Could you check a few things on this drawing? It's one solid part, dimensions in mm from its lowest x, y, z. Give positions to 0.01 mm unless a question says otherwise; leave off trailing zeros. Order: outer loops, then holes, each group sorted by start corner. A loop starts at its lowest first (then second) coordinate and runs counter-clockwise, first axis right, second up. Notation, with made-up numbers: M 16,36 L 43,36 A10 ccw 43,45 Z; hole C 26.5,20 d10. An arc over 180 degrees is marked long. Use one line per item in the form item = value.
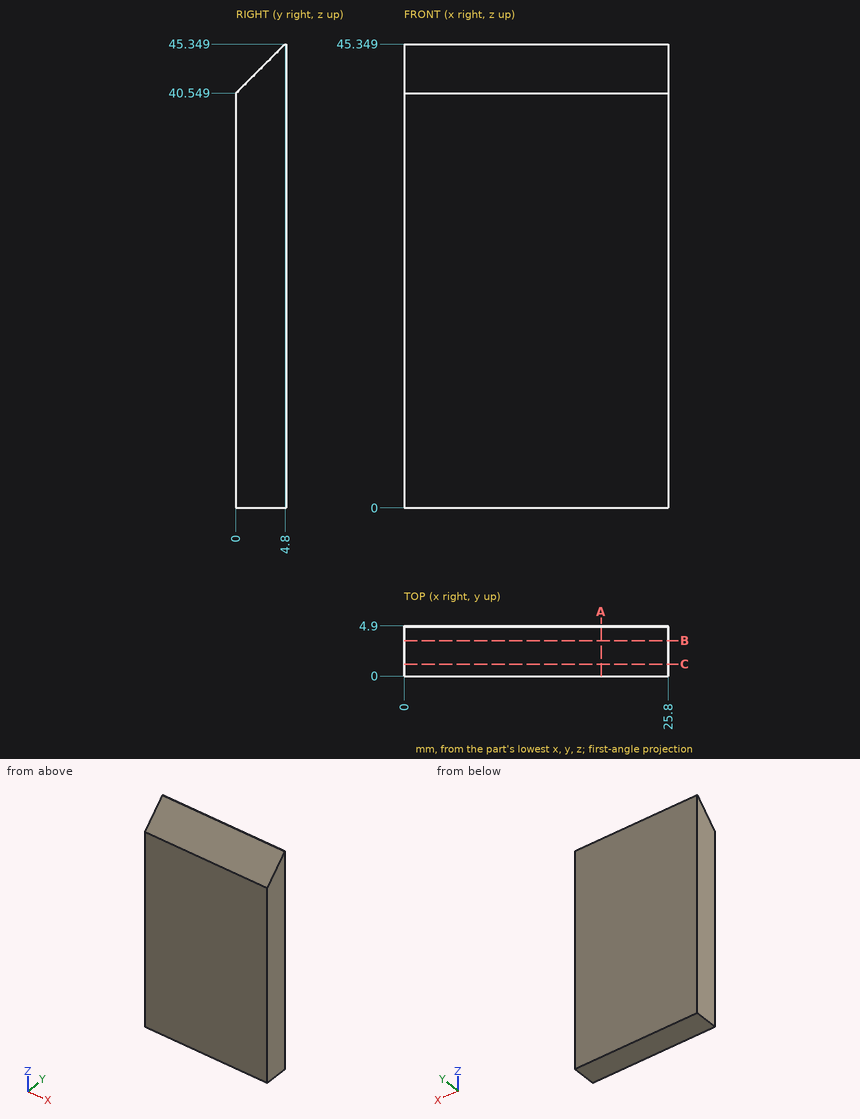
Q1. I want a section at A-A on x = 19.25. Write out the boundary of the cut face in (y, z), then the cut area to 3 significant figures.
Found:
outline = M 0,0 L 4.9,0 L 4.9,45.35 L 4.8,45.35 L 0,40.55 Z
area = 211 mm²
Q2. I want a section at C-C on y = 1.15. Write out the boundary of the cut face in (x, z), then the cut area to 3 significant figures.
Found:
outline = M 0,0 L 25.8,0 L 25.8,41.7 L 0,41.7 Z
area = 1,080 mm²
Q3. I want a section at B-B on y = 3.45. Write out the boundary of the cut face in (x, z), then the cut area to 3 significant figures.
Found:
outline = M 0,0 L 25.8,0 L 25.8,44 L 0,44 Z
area = 1,140 mm²
Q4. I need wall thicknesses on L1, parallel to Z at x = 10.5, y = 2.9; L2, parallel to Z at x = 19.75, y = 1.8. Which ranges of each line are inside material? Lowest first, please.
Found:
L1 = 0 to 43.45
L2 = 0 to 42.35
